Autodesk Inventor part; units mm, degrees
ref_plane "YZ Plane" through (0, 0, 0) normal (1, 0, 0) x (0, 1, 0)
ref_plane "XZ Plane" through (0, 0, 0) normal (0, 1, 0) x (-1, 0, 0)
ref_plane "XY Plane" through (0, 0, 0) normal (0, 0, 1) x (1, 0, 0)
sketch "Sketch1" plane through (0, 0, 0) normal (0, 0, 1) x (1, 0, 0)
  circle A0 centre (0, 0) radius 17.5
  line L0 (-15.1554, -8.75) -> (-13.6554, -11.3481)
  line L1 (-15.1554, -8.75) -> (-16.6554, -6.1519)
  line L2 (0, 0) -> (0, -17.5)
  line L3 (0, 0) -> (15.1554, -8.75)
  line L4 (0, 0) -> (17.5, 0) construction
  line L5 (0, 0) -> (17.5, 0) construction
  line L6 (0, 17.5) -> (0, -17.5)
  line L7 (-15.1554, -8.75) -> (0, 0)
  line L8 (0, -17.5) -> (3, -17.5)
  line L9 (3, -17.5) -> (3, -20.5)
  line L10 (-3, -17.5) -> (0, -17.5)
  line L11 (-3, -17.5) -> (-3, -14)
  line L12 (-3, -10.5) -> (3, -10.5)
  line L13 (3, -10.5) -> (3, -17.5)
  arc A1 (-3, -10.5) -> (-9.5308, -14.9804) centre (-3, -17.5) ccw
  arc A2 (-13.6554, -11.3481) -> (-9.5308, -14.9804) centre (0, 0) ccw
  line L14 (-16.6554, -6.1519) -> (-20.9856, -8.6519)
  line L15 (-20.9856, -8.6519) -> (-19.4856, -11.25)
  arc A3 (-19.4856, -11.25) -> (-3, -22.2991) centre (0, 0) ccw
  line L16 (-3, -14) -> (-3, -22.2991)
  point P0 (0, -10.5)
  point P1 (-3, -17.2409)
  point P2 (3, -17.2409)
  point P3 (-9.4329, -14.7401)
  point P4 (-3, -17.2409)
  dimension "d0" = 35
  dimension "d1" = 3
  dimension "d3" = 3
  dimension "d4" = 330
  dimension "d6" = 35
  dimension "d8" = 3
  dimension "d9" = 3
  dimension "d29" = 7
  dimension "d30" = 6
  dimension "d32" = 5
  dimension "d33" = 3
extrude "Extrusion1" add sketch "Sketch1" along normal blind 12 contours L0 A2 A1 A0 L11 L16 A3 L15 L14 L1 | L13 L8 A0 | A0 L2 L12 L13 | A1 L12 L2 A0 | L10 L11 A0
sketch "Sketch2" plane through (-16.6554, -6.1519, 12) normal (0.866, 0.5, 0) x (0, 0, -1)
  line L0 (0, 0) -> (0, -3)
  line L1 (12, -6) -> (0, -6)
  line L2 (0, -3) -> (12, -3)
  line L3 (0, -3) -> (3, -3)
  line L4 (3, -3) -> (9, -3)
  circle A0 centre (3, -3) radius 1.5
  circle A1 centre (9, -3) radius 1.5
  dimension "d14" = 3
  dimension "d15" = 3
  dimension "d16" = 6
  dimension "d17" = 3
  dimension "d18" = 3
extrude "Extrusion2" cut sketch "Sketch2" against normal blind 12
sketch "Sketch3" plane through (-3, -17.5, 0) normal (0, -1, 0) x (1, 0, 0)
  line L0 (6, 12) -> (0, 12)
  line L1 (3, 0) -> (3, 3)
  line L2 (3, 3) -> (3, 9)
  circle A0 centre (3, 3) radius 1.5
  circle A1 centre (3, 9) radius 1.5
  dimension "d23" = 3
  dimension "d24" = 6
  dimension "d25" = 3
  dimension "d26" = 3
extrude "Extrusion3" cut sketch "Sketch3" against normal blind 12
fillet "Fillet1" radius 2 1 edges at (-3, -22.2991, 6)
properties part number "acopleV2" material "Iron, Ductile"
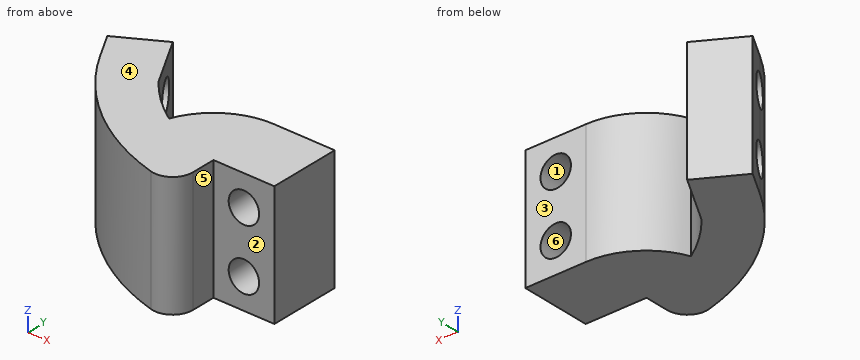
Could you check a few things on this model? Use its own coordinates, in mm. Face numbers are marked on the shaded views. A direction names the side the tool comes from. Give positions to 0.01 mm unless a question says otherwise; leave off trailing zeros. Order: outer loops, then holes, each group sorted by start corner. A loop starts at its lowest first (then second) coordinate and runs counter-clockwise, first axis right, second up.
Q1. Suppose I cut it at B-B, the plane y = -14.25. Write out the boundary of the cut face in (x, z).
Q2. Suppose I cut it at A-A, the plane x = 0. Write out the boundary of the cut face in (y, z), and give its area (3 significant figures).
Q3. I'm going to push flat-ended pins straight in: P1, Ø1.8, axis at x = 0, z = 9, coming from the -Y side; P2, Ø5, axis at x = 1.5, z = 5, coming from the +Y side; P3, Ø1.5, axis at y = -10.5, z = 10.5, coming from the -X side; P4, Ø2.5, axis at y = -19, z = 4.5, coming from the +X side. Where does each tip first touch, or does it pass through?
Q4. Suppose I cut it at D-D, the plane z = 2. Write out the boundary of the cut face in (x, y), and give its area (3 significant figures).
Q5. If I drill on line 1 along Z through (x, y) = (0, -15.75); line 2 along X through (y, z) = (-14.25, 9); line 3 along X through (y, z) = (-13, 3), over which ranges is the centre line in solid material (lowest first)?
Q6. For the marked faces 1, 2 and 3, which set-ups out of +Z, -Z, +X, -X, +Y, -Y let a thin tool reach every point of the face, with its end or its side?
Q7. We'd pull the mould along Z, two halves only. Please class the marked faces 4, 5 and 6: +Z half, -Z half, draft (parallel to the pull), parting line (faces both ways), or undercut.
Q8. Suppose I cut it at C-C, the plane z = 11. Write out the boundary of the cut face in (x, y).
Solution:
1. outline: (-17.41, 0) - (-10.59, 0) - (-10.59, 12) - (-17.41, 12) - close; (-9.2, 0) - (3, 0) - (3, 12) - (-9.2, 12) - close; hole circle Ø3 at (0, 3); hole circle Ø3 at (0, 9)
2. outline: (-17.5, 0) - (-10.5, 0) - (-10.5, 1.5) - (-17.5, 1.5) - close; (-17.5, 4.5) - (-10.5, 4.5) - (-10.5, 7.5) - (-17.5, 7.5) - close; (-17.5, 10.5) - (-10.5, 10.5) - (-10.5, 12) - (-17.5, 12) - close
2. area: 42.0 mm2
3. P1: passes through
3. P2: stops at y = -10.5
3. P3: stops at x = -20.35
3. P4: stops at x = -3
4. outline: (-20.99, -8.65) - (-20.04, -10.28) - (-15.71, -7.78) - (-16.66, -6.15) - close; (-18.9, -12.2) arc R22.5 ccw to (-5.49, -21.82) arc R2 ccw to (-3, -19.88) - (-3, -17.5) - (-1.12, -17.5) - (-1.12, -10.5) - (-3, -10.5) arc R7 ccw to (-9.53, -14.98) arc R17.75 cw to (-13.66, -11.35) - (-14.6, -9.72) - close; (1.12, -17.5) - (3, -17.5) - (3, -10.5) - (1.12, -10.5) - close
4. area: 146 mm2
5. line 1: z = 0 to 1.5, 4.5 to 7.5, 10.5 to 12
5. line 2: x = -17.41 to -10.59, -9.2 to -1.5, 1.5 to 3
5. line 3: x = -18.36 to -12.09, -8.36 to -1.5, 1.5 to 3
6. face 1: +Y, -Y
6. face 2: +Z, -Z, +X, -Y
6. face 3: +Z, -Z, +X, +Y
7. face 4: +Z half
7. face 5: draft
7. face 6: undercut
8. outline: (-20.99, -8.65) - (-19.49, -11.25) arc R22.5 ccw to (-5.49, -21.82) arc R2 ccw to (-3, -19.88) - (-3, -17.5) - (3, -17.5) - (3, -10.5) - (-3, -10.5) arc R7 ccw to (-9.53, -14.98) arc R17.75 cw to (-13.66, -11.35) - (-16.66, -6.15) - close
